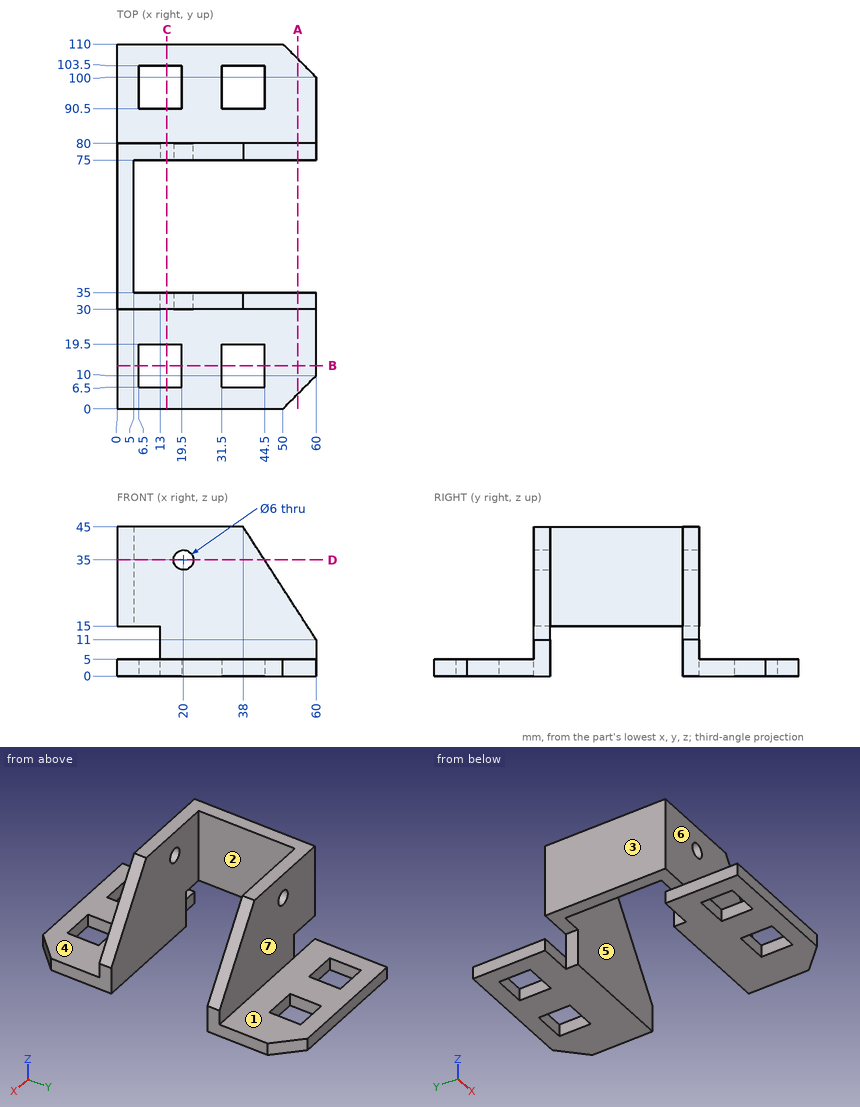
Geometry check sheet. Reference: drawing and pictorial views, mm from the part's lowest x, y, z. A direction names the side the tool comes from. Coordinates: 2 decimals unless noted, no trailing zeros. Order: outer loops, then holes, each group sorted by start corner. A loop starts at its lowest first (then second) coordinate and runs counter-clockwise, first axis right, second up.
Item 1: Release check for a two-part mould opening along Y. For the marked faces 4, 5, 6 and 7 record: +Y half, -Y half, draft (parallel to the pull), parting line (faces both ways), or undercut.
Filled in:
face 4: draft
face 5: undercut
face 6: -Y half
face 7: +Y half
Item 2: Material ranges on L1, parallel to Y at x = 27.5, z = 34.5; L2, parallel to Y at x = 30, z = 4; L3, parallel to X at y = 14, z = 3, recorded low to high.
Filled in:
L1: y = 30 to 35, 75 to 80
L2: y = 0 to 35, 75 to 110
L3: x = 0 to 6.5, 19.5 to 31.5, 44.5 to 60
Item 3: Section check D-D, the plane z = 35. Enter the section's corners in (x, y).
Filled in:
outline: (0, 30) - (17, 30) - (17, 35) - (5, 35) - (5, 75) - (17, 75) - (17, 80) - (0, 80) - close; (23, 30) - (44.47, 30) - (44.47, 35) - (23, 35) - close; (23, 75) - (44.47, 75) - (44.47, 80) - (23, 80) - close
Item 4: Section check A-A, the plane x = 54.5. Enter the section's corners in (y, z), then the cut area to 3 significant figures.
Filled in:
outline: (4.5, 0) - (35, 0) - (35, 19.5) - (30, 19.5) - (30, 5) - (4.5, 5) - close; (75, 0) - (105.5, 0) - (105.5, 5) - (80, 5) - (80, 19.5) - (75, 19.5) - close
area: 450 mm2
Item 5: Section check C-C, the plane x = 15. Enter the section's corners in (y, z).
Filled in:
outline: (0, 0) - (6.5, 0) - (6.5, 5) - (0, 5) - close; (19.5, 0) - (35, 0) - (35, 45) - (30, 45) - (30, 5) - (19.5, 5) - close; (75, 0) - (90.5, 0) - (90.5, 5) - (80, 5) - (80, 45) - (75, 45) - close; (103.5, 0) - (110, 0) - (110, 5) - (103.5, 5) - close
Item 6: Section check B-B, the plane y = 13. Enter the section's corners in (x, z), then the cut area to 3 significant figures.
Filled in:
outline: (0, 0) - (6.5, 0) - (6.5, 5) - (0, 5) - close; (19.5, 0) - (31.5, 0) - (31.5, 5) - (19.5, 5) - close; (44.5, 0) - (60, 0) - (60, 5) - (44.5, 5) - close
area: 170 mm2
Item 7: Depth check by flat-ended pin: pin 1 (12 mm diameter, centred on y = 74, z = 26.5, fed in from +X); pin 2 (1.5 mm diameter, centred on y = 76.5, z = 38.5, fed in from +X); pin 3 (10 mm diameter, centred on x = 47.5, y = 31, fed in from +Z). Enter the tip coordinate at first touch or a pass-through.
Filled in:
pin 1: stops at x = 53.8
pin 2: stops at x = 42.69
pin 3: stops at z = 38.05
Item 8: Access from +Z, -Z, +X, -X, +Y, -Y to the whole of each face (thin tool, end or side, straight path). Record for the marked faces 1, 2 and 3.
Filled in:
face 1: +Z, +X, -X, +Y
face 2: +Z, -Z, +X
face 3: +Z, -Z, -X, +Y, -Y
